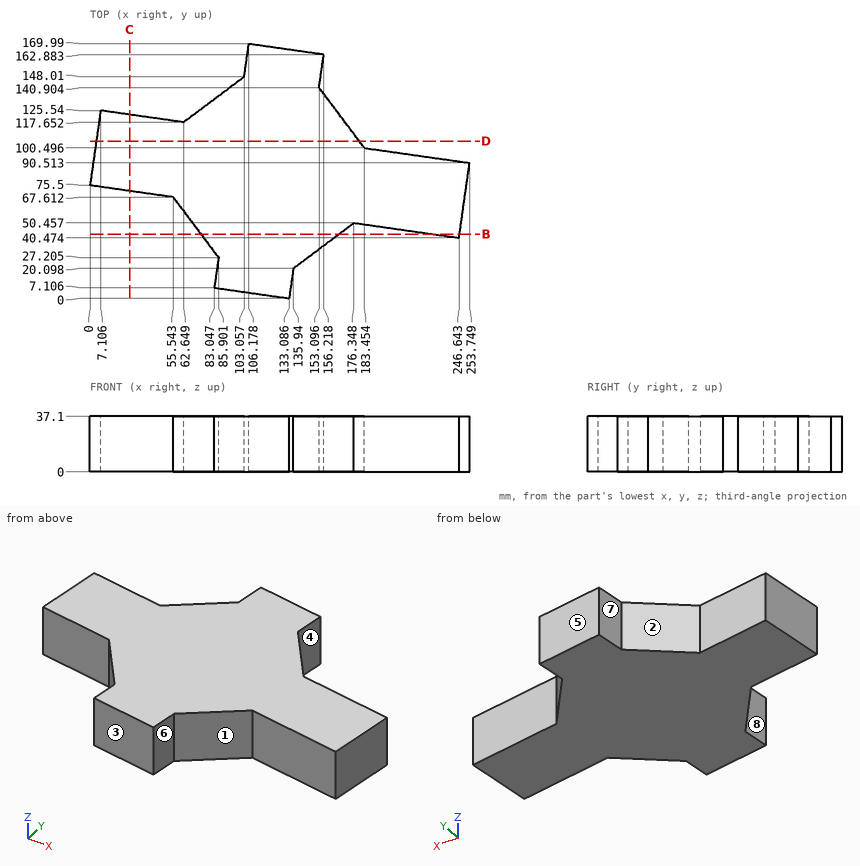
Geometry check sheet. Reference: drawing and pictorial views, mm from the part's lowest x, y, z. A direction names the side the tool comes from. Round coordinates to 2 decimals unless told otherwise and drop trailing zeros. Loops run counter-clockwise (first coordinate to the right, second up) from the corner with the lowest first, then second, coordinate; pieces in that order, holes last.
1. Sectioned sample at B-B on y = 43. Record the boundary of the cut face in (x, z) (1 decimal), and give its area (3 significant figures).
2. Mould release check, pull along Y, two halves, no side actions. Record for the marked faces 6, 7 and 8: released by +Y, released by -Y, zero draft, split by the parting line, or undercut.
3. Scan lines: probe 1 along Y at (x, z) = (15, 30); probe 2 along Y at (x, z) = (228, 33); probe 3 along X at (y, z) = (87, 32). Record each from-to range of solid material in increasing order.
4. Sectioned sample at C-C on x = 26.5. Record the boundary of the cut face in (y, z) (1 decimal).
5. Gauge pin test, flat ends, axial feed: pin 1 Ø1 at (y, z) = (100, 21) entering from -X; pin 2 Ø1.5 at (y, z) = (80, 16) entering from +X; pin 3 Ø8 at (y, z) = (76.5, 30.5) entering from -X. Record the tip position at first contact, or that the pin passes through.
6. Sectioned sample at D-D on y = 105. Record the boundary of the cut face in (x, z).
7. Set-up check for the marked faces 1, 2, 3, 4 and 5: record each of +Z, -Z, +X, -X, +Y, -Y from which the full face is reachable in a straight line by a thin tool's end or side.
Recorded:
1. outline: (74, 0) - (166.4, 0) - (166.4, 37.1) - (74, 37.1) - close; (228.9, 0) - (247, 0) - (247, 37.1) - (228.9, 37.1) - close
1. area: 4,100 mm2
2. face 6: released by -Y
2. face 7: released by +Y
2. face 8: undercut
3. probe 1: y = 73.37 to 124.42
3. probe 2: y = 43.12 to 94.17
3. probe 3: x = 1.63 to 253.25
4. outline: (71.7, 0) - (122.8, 0) - (122.8, 37.1) - (71.7, 37.1) - close
5. pin 1: stops at x = 3.41
5. pin 2: stops at x = 252.36
5. pin 3: stops at x = 0
6. outline: (4.19, 0) - (180.07, 0) - (180.07, 37.1) - (4.19, 37.1) - close
7. face 1: +Z, -Z, -Y
7. face 2: +Z, -Z, +Y
7. face 3: +Z, -Z, -X, -Y
7. face 4: +Z, -Z, +X
7. face 5: +Z, -Z, +X, +Y
